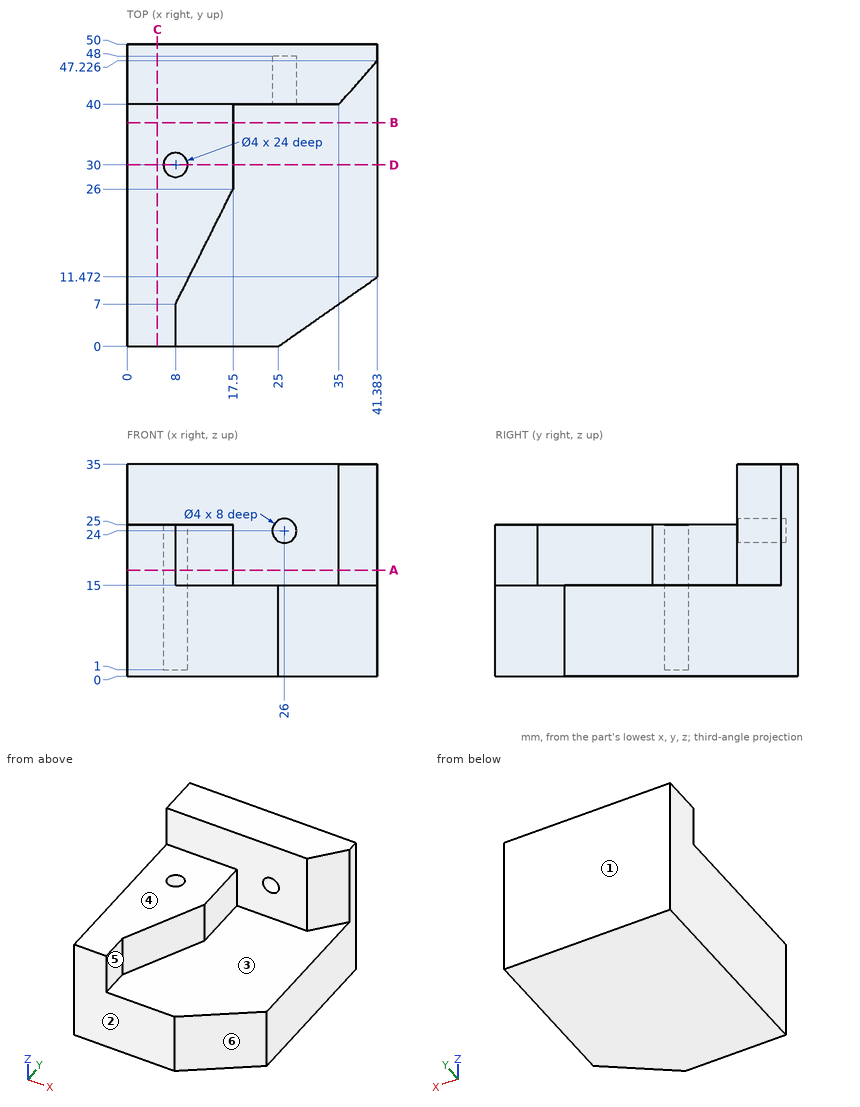
Geometry: see drawing. Coordinates: mm, zero at the bounding-box minimum. A direction names the side the tool comes from. Give positions to 0.01 mm unless a question says otherwise; leave off trailing zeros. Loops run counter-clockwise (first coordinate to the right, second up) from the corner with the lowest first, then second, coordinate; pieces in that order, holes last. Notation, with made-up numbers: M 14,-40 L 18,-40 A24 ccw 18,-15 Z; hole C -0.5,6 d1. An arc over 180 degrees is marked long. Use one line per item in the form item = value.
1. Reachability of the marked faces 4, 5 and 6 from +Z, -Z, +X, -X, +Y, -Y: full face, straight path, thin tool, end or side. Return the list, or none.
Numbers:
face_4 = +Z, +X, -X, -Y
face_5 = +Z, +X, -Y
face_6 = +Z, -Z, +X, -Y
2. Pull-direction query (Y, two-part tool) for the marked faces 1, 2 and 3; classes: released by +Y, released by -Y, zero draft, split by the parting line, or undercut.
Numbers:
face_1 = released by +Y
face_2 = released by -Y
face_3 = zero draft
3. Section query B-B, the plane y = 37. Return the cut outline in (x, z).
Numbers:
outline = M 0,0 L 41.38,0 L 41.38,15 L 17.5,15 L 17.5,25 L 0,25 Z
4. Section query D-D, the plane y = 30. Return the cut outline in (x, z).
Numbers:
outline = M 0,0 L 41.38,0 L 41.38,15 L 17.5,15 L 17.5,25 L 10,25 L 10,1 L 6,1 L 6,25 L 0,25 Z
5. Section query A-A, the plane z = 17.5. Return the cut outline in (x, y).
Numbers:
outline = M 0,0 L 8,0 L 8,7 L 17.5,26 L 17.5,40 L 35,40 L 41.38,47.23 L 41.38,50 L 0,50 Z; hole C 8,30 d4
6. Line query: L1, parallel to Z at x = 26, y = 43.75; L2, parallel to X at y = 30, z = 6; L3, parallel to Y at x = 8, z = 13. Output: solid intervals per line, ascending.
Numbers:
L1 = 0 to 22, 26 to 35
L2 = 0 to 6, 10 to 41.38
L3 = 0 to 28, 32 to 50
7. First-contact query: pin 1 (3 mm diameter, centred on x = 9, y = 29, fed in from +Z); pin 2 (1.5 mm diameter, centred on y = 23.5, z = 23, fed in from +X) (1 decimal); pin 3 (1.2 mm diameter, centred on x = 26.5, z = 25, fed in from -Y). Flat tips, straight axial feed; report the tip coordinate or a pass-through.
Numbers:
pin_1 = 25
pin_2 = 16.6
pin_3 = 48
8. Section query C-C, the plane x = 5. Return the cut outline in (y, z), and give its area (3 significant figures).
Numbers:
outline = M 0,0 L 50,0 L 50,35 L 40,35 L 40,25 L 0,25 Z
area = 1,350 mm²
